The listing builds one solid part. Answer for the finished solid, in the listing's coordinates (mm). A direction names the side the tool comes from. Give positions to 0.01 mm unless a question says otherwise; leave off trailing zeros. Loops run counter-clockwise (first coordinate to the right, second up) from the corner with the lowest first, then second, coordinate; pieces in that order, holes last. Notation, with made-up numbers: (-26, 28) - (22, 28) arc R29 ccw to (22, 62) - close; hole circle Ø3 at (80, 43). An arc over 180 degrees is marked (long way). Answer as CSV lines item,"result". Start each with the question number.
1) Flat-ended cylindrical pins translate along their axes: pin 1 (11 mm diameter, centred on x = 0, z = 19.7, fed in from +Y); pin 2 (0.9 mm diameter, centred on x = 5.5, y = 1.5, fed in from +Z). Find the tip coordinate at first contact, or state that the pin passes through.
2) Find the intervals of material crossed by line 1 along X through (y, z) = (2.05, 50.5); line 2 along X through (y, z) = (2.3, 52.5); line 3 along Z through (x, y) = (-47, 1), in increasing order.
3) A cutting plane is placed at B-B (y = 1.65). Determine the outline of the cut face in (x, z) (3 decimals), and give its area (3 significant figures).
4) For faces 5 (the face through (2.703, 1.479, 28.283)), 6 (the face through (0, 1, 43.199)), determine the directions among +Z, -Z, +X, -X, +Y, -Y from which every point of the face is accessible in a straight line to the end or side of a thin tool.
5) For a pull along X with two mould halves and no side action, classify faces 1 (the face through (19.975, 1.479, 44.06)), 2 (the face through (-34.455, 1.479, 10.623)), 3 (the face through (-1, 3, 29)), 4 (the face through (35.085, 1.479, 11.519)) as pulls with the +X half, pulls with the -X half, needs draft (parallel to the pull), parting line crosses it, or undercut.
6) A cutting plane is placed at C-C (z = 57.5). Determine the outline of the cut face in (x, y), and give its area (3 significant figures).
7) A cutting plane is placed at D-D (x = 45). Determine the outline of the cut face in (y, z).
8) A cutting plane is placed at A-A (x = 0). Determine the outline of the cut face in (y, z).
```python
from build123d import *

# Parameters (mm, degrees)
SKETCH1_R           = 9
SKETCH1_R_2         = 3.175
BOSS_EXTRUDE1_DEPTH = 3


with BuildPart() as part:
    # Sketch1 → Boss-Extrude1 (new body)
    with BuildSketch(Plane(origin=(0, 0, 0), x_dir=(1, 0, 0), z_dir=(0, 1, 0))):
        with BuildLine():
            Line((-12.270437376, 20.928622154), (-57.270437376, -43.071377846))
            ThreePointArc((-57.270437376, -43.071377846), (-53.677181673, -63.93449063), (-32.7997143, -60.425599405))
            Line((-32.7997143, -60.425599405), (-22.871154784, -46.544858311))
            ThreePointArc((-22.871154784, -46.544858311), (-20.022657317, -44.084488856), (-16.364335743, -43.199029126))
            Line((-16.364335743, -43.199029126), (16.364335743, -43.199029126))
            ThreePointArc((16.364335743, -43.199029126), (20.022657317, -44.084488856), (22.871154784, -46.544858311))
            Line((22.871154784, -46.544858311), (32.7997143, -60.425599405))
            ThreePointArc((32.7997143, -60.425599405), (53.677181673, -63.93449063), (57.270437376, -43.071377846))
            Line((57.270437376, -43.071377846), (12.270437376, 20.928622154))
            ThreePointArc((12.270437376, 20.928622154), (0, 27.300970874), (-12.270437376, 20.928622154))
        make_face()
        with Locations(Location((0, -19.699029126, 0), (0, 0, 270))):
            Circle(SKETCH1_R, mode=Mode.SUBTRACT)
        with Locations(Location((-45, -51.699029126, 0), (0, 0, 270))):
            Circle(SKETCH1_R_2, mode=Mode.SUBTRACT)
        with Locations(Location((0, 12.300970874, 0), (0, 0, 270))):
            Circle(SKETCH1_R_2, mode=Mode.SUBTRACT)
        with Locations(Location((45, -51.699029126, 0), (0, 0, 270))):
            Circle(SKETCH1_R_2, mode=Mode.SUBTRACT)
    extrude(amount=BOSS_EXTRUDE1_DEPTH)


solid = part.part
```
Ans:
1,pin 1,"through"
1,pin 2,"z = 43.2"
2,line 1,"-59.95 to -47.94, -42.06 to -25.7, 25.7 to 42.06, 47.94 to 59.95"
2,line 2,"-59.98 to -48.07, -41.93 to -27.13, 27.13 to 41.93, 48.07 to 59.98"
2,line 3,"28.46 to 49.23, 54.16 to 66.57"
3,outline,"(-57.27, 43.071) - (-12.27, -20.929) arc R15 ccw to (12.27, -20.929) - (57.27, 43.071) arc R15 ccw to (32.8, 60.426) - (22.871, 46.545) arc R8 cw to (16.364, 43.199) - (-16.364, 43.199) arc R8 cw to (-22.871, 46.545) - (-32.8, 60.426) arc R15 ccw to start; hole circle Ø6.35 at (-45, 51.699); hole circle Ø18 at (0, 19.699); hole circle Ø6.35 at (0, -12.301); hole circle Ø6.35 at (45, 51.699)"
3,area,"5,560 mm2"
4,face 5,"+Y, -Y"
4,face 6,"+Z, +Y, -Y"
5,face 1,"undercut"
5,face 2,"pulls with the -X half"
5,face 3,"needs draft"
5,face 4,"pulls with the +X half"
6,outline,"(-58.83, 0) - (-30.71, 0) - (-30.71, 3) - (-58.83, 3) - close; (30.71, 0) - (58.83, 0) - (58.83, 3) - (30.71, 3) - close"
6,area,"169 mm2"
7,outline,"(0, 25.62) - (3, 25.62) - (3, 48.52) - (0, 48.52) - close; (0, 54.87) - (3, 54.87) - (3, 66.7) - (0, 66.7) - close"
8,outline,"(0, -27.3) - (3, -27.3) - (3, -15.48) - (0, -15.48) - close; (0, -9.13) - (3, -9.13) - (3, 10.7) - (0, 10.7) - close; (0, 28.7) - (3, 28.7) - (3, 43.2) - (0, 43.2) - close"
